Could you check a few things on this model? Use its own coordinates, in mm. Round coordinates to 2 decimals unless told otherwise and drop trailing zeros. Loops run counter-clockwise (first coordinate to the right, second up) from the corner with the lowest first, then second, coordinate; pieces in that order, holes last.
Autodesk Inventor part; units mm, degrees
ref_plane "YZ Plane" through (0, 0, 0) normal (1, 0, 0) x (0, 1, 0)
ref_plane "XZ Plane" through (0, 0, 0) normal (0, 1, 0) x (-1, 0, 0)
ref_plane "XY Plane" through (0, 0, 0) normal (0, 0, 1) x (1, 0, 0)
sketch "スケッチ1" plane through (0, 0, 0) normal (0, 0, 1) x (1, 0, 0)
  point P0 (0, 0)
sketch "スケッチ2" plane through (0, 0, 0) normal (1, 0, 0) x (0, 1, 0)
  circle A0 centre (0, 0) radius 12.5
  circle A1 centre (0, 0) radius 4
  dimension "d0" = 25
  dimension "d1" = 8
extrude "押し出し1" add sketch "スケッチ2" along normal blind 6
sketch "スケッチ3" plane through (6, 0, 0) normal (1, 0, 0) x (0, 0, -1)
  circle A0 centre (0, 0) radius 8.5 construction
  circle A1 centre (0, 8.5) radius 1.6
  circle A2 centre (-8.5, 0) radius 1.6
  circle A3 centre (0, -8.5) radius 1.6
  circle A4 centre (8.5, 0) radius 1.6
  dimension "d4" = 17
  dimension "d5" = 3.2
  dimension "d6" = 3.2
  dimension "d7" = 3.2
  dimension "d8" = 3.2
hole "穴1" at (6, 8.5, 0) at (6, 0, 8.5) at (6, -8.5, 0) at (6, 0, -8.5) direction (-1, 0, 0) diameter 3.2 end through all
properties part number "NHK_t0_7"
Item 1: If I drill on line 1 along Z through (x, y) = (4.55, 0); line 2 along Z through (x, y) = (3.05, -8.5); line 3 along Z through (x, y) = (0.7, -1.25), over which ranges is the centre line in solid material (lowest first)?
Results list:
line 1: z = -12.5 to -10.1, -6.9 to -4, 4 to 6.9, 10.1 to 12.5
line 2: z = -9.17 to -1.6, 1.6 to 9.17
line 3: z = -12.44 to -9.5, -7.5 to -3.8, 3.8 to 7.5, 9.5 to 12.44
Item 2: If we section it at C-C, the plane z = -8: Please give me the cut outline in (x, y), then the cut area to 3 significant figures.
Results list:
outline: (0, -9.6) - (6, -9.6) - (6, -1.52) - (0, -1.52) - close; (0, 1.52) - (6, 1.52) - (6, 9.6) - (0, 9.6) - close
area: 97.0 mm2
Item 3: We'd pull the mould along Y, two halves only. Please class faces 1 (the cylindrical face through (2.958, 11.923, -3.755)), 2 (the cylindrical face through (2.958, -0.867, 3.905)), 3 (the flat face through (6, -3, 3)): released by +Y, released by -Y, zero draft, split by the parting line, or undercut.
Results list:
face 1: split by the parting line
face 2: undercut
face 3: zero draft
Item 4: If we section it at D-D, the plane y = 8.5: Please give me the cut outline in (x, z).
Results list:
outline: (0, -9.17) - (6, -9.17) - (6, -1.6) - (0, -1.6) - close; (0, 1.6) - (6, 1.6) - (6, 9.17) - (0, 9.17) - close
Item 5: If we section it at A-A, the plane y = 0: Please give me the cut outline in (x, z).
Results list:
outline: (0, -12.5) - (6, -12.5) - (6, -10.1) - (0, -10.1) - close; (0, -6.9) - (6, -6.9) - (6, -4) - (0, -4) - close; (0, 4) - (6, 4) - (6, 6.9) - (0, 6.9) - close; (0, 10.1) - (6, 10.1) - (6, 12.5) - (0, 12.5) - close
Item 6: Will these pins go through, and if not, where does the flat tip stop? pin 1 (3 mm diameter, centred on y = 6.5, z = -6.5, fed in from -X); pin 2 (2.5 mm diameter, centred on y = 0, z = 8.5, fed in from +X); pin 3 (1.5 mm diameter, centred on x = 2, z = 9.5, fed in from -Y); pin 4 (3 mm diameter, centred on x = 2.5, y = -5, fed in from -Z).
Results list:
pin 1: stops at x = 0
pin 2: passes through
pin 3: stops at y = -8.93
pin 4: stops at z = -12
